Source: CAD feature listing. Evaluate the final solid. Frame: model axes, mm. A direction names the side the tool comes from. Give positions to 0.01 mm unless a question says otherwise; leave off trailing zeros. Order: outer loops, then holes, each group sorted by start corner. A loop starts at its lowest first (then second) coordinate and runs counter-clockwise, first axis right, second up.
from build123d import *

# Parameters (mm, degrees)
SKETCH1_R           = 3.5687
SKETCH1_R_2         = 2
BOSS_EXTRUDE1_DEPTH = 4.191
SKETCH5_R           = 2
SKETCH5_R_2         = 1.143
BOSS_EXTRUDE2_DEPTH = 0.2226
BOSS_EXTRUDE3_START = -1.524
SKETCH6_R           = 0.5334
BOSS_EXTRUDE3_DEPTH = 1.524
BOSS_EXTRUDE4_START = -1.524
BOSS_EXTRUDE4_DEPTH = 1.524


with BuildPart() as part:
    # Sketch1 → Boss-Extrude1 (new body)
    with BuildSketch(Plane.XY.offset(-7.032965862)):
        with Locations((-5.5, 0)):
            Circle(SKETCH1_R)
        with Locations((-5.5, 0)):
            Circle(SKETCH1_R_2, mode=Mode.SUBTRACT)
    extrude(amount=BOSS_EXTRUDE1_DEPTH)

    # Sketch5 → Boss-Extrude2 (add)
    with BuildSketch(Plane.XY.offset(-4.232965862)):
        with Locations((-5.5, 0)):
            Circle(SKETCH5_R)
        with Locations((-5.5, 0)):
            Circle(SKETCH5_R_2, mode=Mode.SUBTRACT)
    extrude(amount=BOSS_EXTRUDE2_DEPTH)

    # Sketch6 → Boss-Extrude3 (add)
    with BuildSketch(Plane.XY.offset(-2.841965862).offset(BOSS_EXTRUDE3_START)):
        with BuildLine():
            Line((-4, -13.25), (-2.68695, -2.195989387))
            ThreePointArc((-2.68695, -2.195989387), (-5.5, -3.5687), (-8.31305, -2.195989387))
            Line((-8.31305, -2.195989387), (-7, -13.25))
            ThreePointArc((-7, -13.25), (-5.5, -14.75), (-4, -13.25))
        make_face()
        with Locations((-5.5, -12.0816)):
            Circle(SKETCH6_R, mode=Mode.SUBTRACT)
        with Locations((-5.5, -13.7834)):
            Circle(SKETCH6_R, mode=Mode.SUBTRACT)
        with Locations((-5.5, -10.3798)):
            Circle(SKETCH6_R, mode=Mode.SUBTRACT)
        with Locations((-5.5, -8.678)):
            Circle(SKETCH6_R, mode=Mode.SUBTRACT)
        with Locations((-5.5, -6.9762)):
            Circle(SKETCH6_R, mode=Mode.SUBTRACT)
        with Locations((-5.5, -5.2744)):
            Circle(SKETCH6_R, mode=Mode.SUBTRACT)
    boss_extrude3 = extrude(amount=BOSS_EXTRUDE3_DEPTH)

    # Mirror1: Boss-Extrude3 across plane
    add(boss_extrude3.mirror(Plane.ZX))

    # Sketch7 → Boss-Extrude4 (add)
    with BuildSketch(Plane.XY.offset(-2.841965862).offset(BOSS_EXTRUDE4_START)):
        with BuildLine():
            Line((-16.036523348, -1.481234859), (-7.695989387, -2.81305))
            ThreePointArc((-7.695989387, -2.81305), (-9.0687, 0), (-7.695989387, 2.81305))
            Line((-7.695989387, 2.81305), (-16.036523348, 1.481234859))
            ThreePointArc((-16.036523348, 1.481234859), (-17.3, 0), (-16.036523348, -1.481234859))
        make_face()
    boss_extrude4 = extrude(amount=BOSS_EXTRUDE4_DEPTH)

    # Mirror2: Boss-Extrude4 across plane
    add(boss_extrude4.mirror(Plane.ZY.offset(5.5)))


solid = part.part
1) Section query B-B on x = -5.5. State how many separate pieces and enclosed holes the cut face has, and give its area (3 significant figures).
Checks:
separate pieces: 14
enclosed holes: 0
area: 28.1 mm2
2) Pull-direction query (Y, two-part tool) for faces 1 (the face through (6.3, 0, -3.6)), 2 (the face through (-5.5, -1.3, -4.01)), 3 (the face through (-5.53, -14.75, -3.61)), 4 (the face through (-1.9, -1, -4.366)); classes: +Y half, -Y half, draft (parallel to the pull), parting line (faces both ways), or undercut.
Checks:
face 1: parting line
face 2: undercut
face 3: -Y half
face 4: draft
3) Section query D-D on z = -6.25. Output: boundary loops of the cut face in (x, y), and give its area (3 significant figures).
Checks:
outline: circle Ø7.14 at (-5.5, 0); hole circle Ø4 at (-5.5, 0)
area: 27.4 mm2
4) Reachability of faces 5 (the face through (-7.1, -1.2, -3.4)), 6 (the face through (-5.5, -1.3, -4.233)), 7 (the face through (-4.99, -6.82, -3.61)) from +Z, -Z, +X, -X, +Y, -Y: full face, straight path, thin tool, end or side. Return the list, or none.
Checks:
face 5: +Z
face 6: -Z
face 7: +Z, -Z
5) Ray query, L1, parallel to Z at x = -9, y = 2.25; L2, parallel to Y at x = -4.25, z = -4.95; L3, parallel to X at y = 7, z = -4.1. Return the intervals inside material, ascending.
Checks:
L1: z = -4.37 to -2.84
L2: y = -3.34 to -1.56, 1.56 to 3.34
L3: x = -7.74 to -6.03, -4.97 to -3.26
6) First-contact query: pin 1 Ø4.5 at (x, y) = (-5.5, 0) entering from -Z; pin 2 Ø1 at (y, z) = (8, -4) entering from +X; pin 3 Ø1.7 at (x, y) = (-5.5, -13.78) entering from -Z. Flat tips, straight axial feed; report the tip coordinate or a pass-through.
Checks:
pin 1: stops at z = -7.03
pin 2: stops at x = -3.32
pin 3: stops at z = -4.37
7) Section query A-A on y = 0. Output: boundary loops of the cut face in (x, z).
Checks:
outline: (-17.3, -4.37) - (-9.07, -4.37) - (-9.07, -7.03) - (-7.5, -7.03) - (-7.5, -4.23) - (-6.64, -4.23) - (-6.64, -4.01) - (-7.5, -4.01) - (-7.5, -2.84) - (-17.3, -2.84) - close; (-4.36, -4.23) - (-3.5, -4.23) - (-3.5, -7.03) - (-1.93, -7.03) - (-1.93, -4.37) - (6.3, -4.37) - (6.3, -2.84) - (-3.5, -2.84) - (-3.5, -4.01) - (-4.36, -4.01) - close
